Job drawing, mm, ordinate dimensions from the low corner. One solid piece. Give positions to 0.01 mm unless a question says otherwise; leave off trailing zeros. Loops run counter-clockwise (first coordinate to the right, second up) from the corner with the lowest first, then second, coordinate; pieces in that order, holes last. Notation, with made-up numbers: (12, 18.5) -> (61, 18.5) arc R16 cw to (61, 39.5) -> close; hole circle Ø5 at (78.25, 33). An arc over 180 degrees is marked (long way). Answer as a JSON object with one key per item and string values. Group by question number.
Q1. Band-saw the part on C-C, the plane z = 90. Write the cut outline in (x, y), plus the area to 3 significant figures.
Q2. Band-saw the part on A-A, the plane y = 0.9. Write the cut outline in (x, z), plus the area to 3 significant figures.
Q3. Band-saw the part on B-B, the plane x = 10.5. Write the cut outline in (y, z), plus the area to 3 significant figures.
Q4. Wall check: probe 1 along X at (y, z) = (3.25, 21); probe 2 along X at (y, z) = (1.6, 90); probe 3 along X at (y, z) = (0.25, 9.5). Give the ranges that are in metal, low to high. Write a range as from..to.
Q5. Drop a flat-ended pin along its axis: pin 1 (1.9 mm diameter, centred on x = 10.5, z = 90, fed in from -Y). Give the stop position or say it passes through.
Q6. Band-saw the part on D-D, the plane z = 21. Write the cut outline in (x, y).
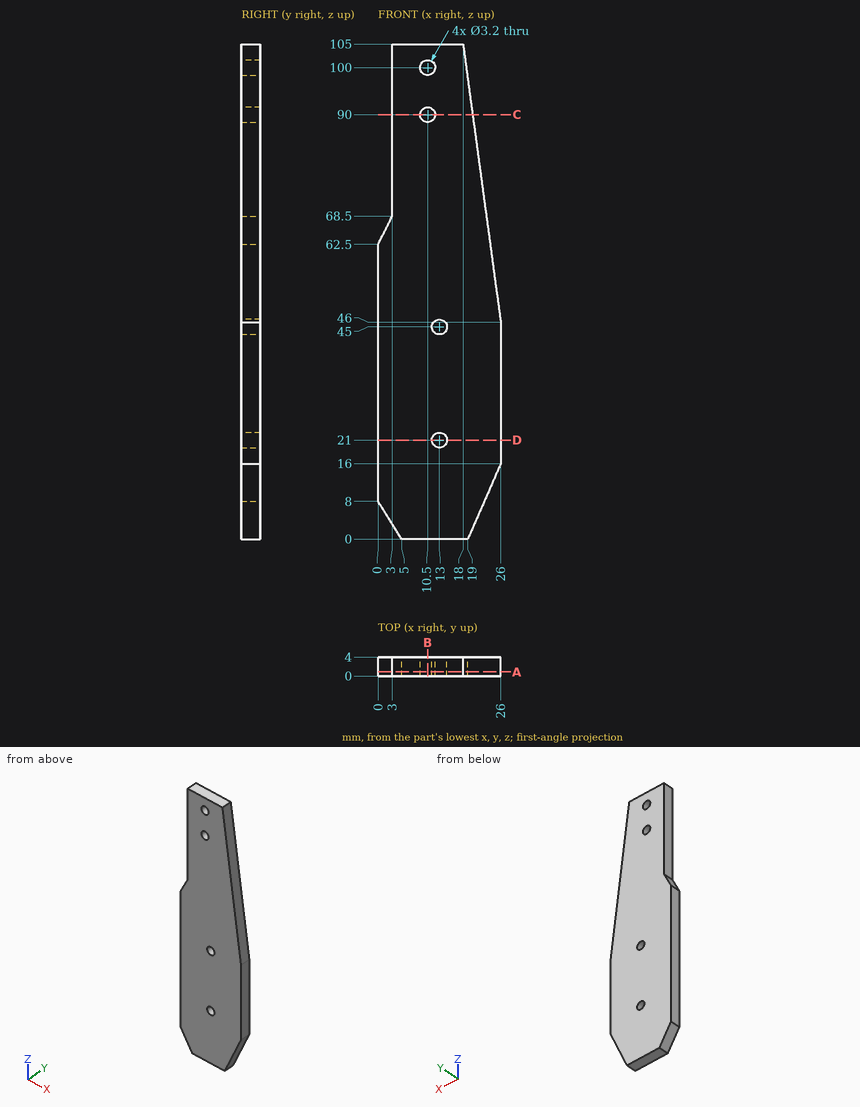
Worked answers:
{
 "1": {"outline": "(3, 0) -> (8.9, 0) -> (8.9, 4) -> (3, 4) -> close; (12.1, 0) -> (20.03, 0) -> (20.03, 4) -> (12.1, 4) -> close", "area": "55.3 mm2"},
 "2": {"outline": "(0, 8) -> (5, 0) -> (19, 0) -> (26, 16) -> (26, 46) -> (18, 105) -> (3, 105) -> (3, 68.5) -> (0, 62.5) -> close; hole circle Ø3.2 at (10.5, 90); hole circle Ø3.2 at (10.5, 100); hole circle Ø3.2 at (13, 21); hole circle Ø3.2 at (13, 45)", "area": "2,270 mm2"},
 "3": {"outline": "(0, 0) -> (4, 0) -> (4, 88.4) -> (0, 88.4) -> close; (0, 91.6) -> (4, 91.6) -> (4, 98.4) -> (0, 98.4) -> close; (0, 101.6) -> (4, 101.6) -> (4, 105) -> (0, 105) -> close", "area": "394 mm2"},
 "4": {"probe 1": "0..11.4, 14.6..26", "probe 2": "3..8.9, 12.1..20.03", "probe 3": "0..23.16"},
 "5": {"pin 1": "through"},
 "6": {"outline": "(0, 0) -> (11.4, 0) -> (11.4, 4) -> (0, 4) -> close; (14.6, 0) -> (26, 0) -> (26, 4) -> (14.6, 4) -> close"}
}
